CAD build for the part. Positions are in the model's coordinates, mm. Face numbers are marked on the shaded views. A direction names the side the tool comes from. Round coordinates to 2 decimals unless told otherwise and drop trailing zeros. Loops run counter-clockwise (first coordinate to the right, second up) from the corner with the lowest first, then second, coordinate; pieces in that order, holes last. Notation, with made-up numbers: (26.5, 27) - (34.5, 27) arc R25 ccw to (34.5, 65) - close; hole circle Ø1 at (81, 88.5). An arc over 180 degrees is marked (long way). One line per question, with ' | ' between items.
```python
from build123d import *

# Parameters (mm, degrees)
SKETCH2_W           = 200
SKETCH2_H           = 100
SKETCH2_W_2         = 190
SKETCH2_H_2         = 90
SKETCH2_W_3         = 65.966934908
SKETCH2_H_3         = 42.5
BOSS_EXTRUDE1_DEPTH = 5
SKETCH4_W           = 200
SKETCH4_H           = 100
SKETCH4_W_2         = 190
SKETCH4_H_2         = 90
BOSS_EXTRUDE2_DEPTH = 90
SKETCH5_W           = 70
SKETCH5_H           = 22.5
CUT_EXTRUDE1_DEPTH  = 90
SKETCH6_W           = 70
SKETCH6_H           = 22.5
CUT_EXTRUDE2_DEPTH  = 90
SKETCH7_W           = 40
SKETCH7_H           = 70
CUT_EXTRUDE3_DEPTH  = 10
SKETCH8_W           = 40
SKETCH8_H           = 70
CUT_EXTRUDE4_DEPTH  = 10
SKETCH9_W           = 40
SKETCH9_H           = 70
CUT_EXTRUDE5_DEPTH  = 10
SKETCH10_R          = 2
CUT_EXTRUDE6_DEPTH  = 10
SKETCH11_R          = 5
CUT_EXTRUDE7_DEPTH  = 150
SKETCH12_R          = 5
CUT_EXTRUDE8_DEPTH  = 10
SKETCH13_R          = 5
CUT_EXTRUDE9_DEPTH  = 10
SKETCH14_R          = 5
CUT_EXTRUDE10_DEPTH = 10
SKETCH16_R          = 0.2
CUT_EXTRUDE11_DEPTH = 10
SKETCH17_W          = 40
SKETCH17_H          = 5
BOSS_EXTRUDE3_DEPTH = 70
SKETCH18_W          = 40
SKETCH18_H          = 5
BOSS_EXTRUDE4_DEPTH = 70


with BuildPart() as part:
    # Sketch2 → Boss-Extrude1 (new body)
    with BuildSketch(Plane.XY):
        Rectangle(SKETCH2_W, SKETCH2_H)
        Rectangle(SKETCH2_W_2, SKETCH2_H_2, mode=Mode.SUBTRACT)
        Polygon((-29.033065092, -2.5), (-29.033065092, -45), (95, -45), (95, 45), (-29.033065092, 45), (-29.033065092, 2.5), (-95, 2.5), (-95, -2.5), align=None)
        with Locations((-62.016532546, -23.75)):
            Rectangle(SKETCH2_W_3, SKETCH2_H_3)
        with Locations((-62.016532546, 23.75)):
            Rectangle(SKETCH2_W_3, SKETCH2_H_3)
    extrude(amount=BOSS_EXTRUDE1_DEPTH)

    # Sketch4 → Boss-Extrude2 (add)
    with BuildSketch(Plane(origin=(0, 0, 0), x_dir=(-1, 0, 0), z_dir=(0, 0, -1))):
        Rectangle(SKETCH4_W, SKETCH4_H)
        Rectangle(SKETCH4_W_2, SKETCH4_H_2, mode=Mode.SUBTRACT)
        Polygon((30, -45), (35, -45), (35, -2.5), (95, -2.5), (95, 2.5), (35, 2.5), (35, 45), (30, 45), (30, 2.5), (-30, 2.5), (-30, 45), (-35, 45), (-35, 2.5), (-95, 2.5), (-95, -2.5), (-35, -2.5), (-35, -45), (-30, -45), (-30, -2.5), (30, -2.5), align=None)
    extrude(amount=BOSS_EXTRUDE2_DEPTH)

    # Sketch5 → Cut-Extrude1 (cut)
    with BuildSketch(Plane.ZY.offset(35)):
        with Locations((-45, 23.75)):
            Rectangle(SKETCH5_W, SKETCH5_H)
    extrude(amount=-CUT_EXTRUDE1_DEPTH, mode=Mode.SUBTRACT)

    # Sketch6 → Cut-Extrude2 (cut)
    with BuildSketch(Plane.ZY.offset(35)):
        with Locations((-45, -23.75)):
            Rectangle(SKETCH6_W, SKETCH6_H)
    extrude(amount=-CUT_EXTRUDE2_DEPTH, mode=Mode.SUBTRACT)

    # Sketch7 → Cut-Extrude3 (cut)
    with BuildSketch(Plane(origin=(0, -2.5, 0), x_dir=(-1, 0, 0), z_dir=(0, -1, 0))):
        with Locations((65, 45)):
            Rectangle(SKETCH7_W, SKETCH7_H)
    extrude(amount=-CUT_EXTRUDE3_DEPTH, mode=Mode.SUBTRACT)

    # Sketch8 → Cut-Extrude4 (cut)
    with BuildSketch(Plane(origin=(0, -2.5, 0), x_dir=(-1, 0, 0), z_dir=(0, -1, 0))):
        with Locations((0, 45)):
            Rectangle(SKETCH8_W, SKETCH8_H)
    extrude(amount=-CUT_EXTRUDE4_DEPTH, mode=Mode.SUBTRACT)

    # Sketch9 → Cut-Extrude5 (cut)
    with BuildSketch(Plane(origin=(0, -2.5, 0), x_dir=(-1, 0, 0), z_dir=(0, -1, 0))):
        with Locations((-65, 45)):
            Rectangle(SKETCH9_W, SKETCH9_H)
    extrude(amount=-CUT_EXTRUDE5_DEPTH, mode=Mode.SUBTRACT)

    # Sketch10 → Cut-Extrude6 (cut)
    with BuildSketch(Plane(origin=(0, 0, -90), x_dir=(-1, 0, 0), z_dir=(0, 0, -1))):
        with Locations((32.5, 0)):
            Circle(SKETCH10_R)
        with Locations((97.5, -47.5)):
            Circle(SKETCH10_R)
        with Locations(Location((97.5, 47.5, 0), (0, 0, 180))):
            Circle(SKETCH10_R)
        with Locations((-97.5, 47.5)):
            Circle(SKETCH10_R)
        with Locations(Location((-32.5, 0, 0), (0, 0, 180))):
            Circle(SKETCH10_R)
        with Locations(Location((-97.5, -47.5, 0), (0, 0, 180))):
            Circle(SKETCH10_R)
    extrude(amount=-CUT_EXTRUDE6_DEPTH, mode=Mode.SUBTRACT)

    # Sketch11 → Cut-Extrude7 (cut)
    with BuildSketch(Plane(origin=(0, -50, 0), x_dir=(-1, 0, 0), z_dir=(0, -1, 0))):
        with Locations(Location((60, 45, 0), (0, 0, 90))):
            Circle(SKETCH11_R)
        with Locations(Location((-60, 45, 0), (0, 0, 90))):
            Circle(SKETCH11_R)
    extrude(amount=-CUT_EXTRUDE7_DEPTH, mode=Mode.SUBTRACT)

    # Sketch12 → Cut-Extrude8 (cut)
    with BuildSketch(Plane.ZY.offset(100)):
        with Locations(Location((-42.5, -35, 0), (0, 0, 270))):
            Circle(SKETCH12_R)
    extrude(amount=-CUT_EXTRUDE8_DEPTH, mode=Mode.SUBTRACT)

    # Sketch13 → Cut-Extrude9 (cut)
    with BuildSketch(Plane(origin=(100, 0, 0), x_dir=(0, 0, -1), z_dir=(1, 0, 0))):
        with Locations(Location((42.5, -35, 0), (0, 0, 270))):
            Circle(SKETCH13_R)
    extrude(amount=-CUT_EXTRUDE9_DEPTH, mode=Mode.SUBTRACT)

    # Sketch14 → Cut-Extrude10 (cut)
    with BuildSketch(Plane.XY.offset(5)):
        with Locations((-70, -20)):
            Circle(SKETCH14_R)
        with Locations((70, -20)):
            Circle(SKETCH14_R)
    extrude(amount=-CUT_EXTRUDE10_DEPTH, mode=Mode.SUBTRACT)

    # Sketch16 → Cut-Extrude11 (cut)
    with BuildSketch(Plane.XZ.offset(50)):
        with Locations(Location((90, -5, 0), (0, 0, 270))):
            Circle(SKETCH16_R)
        with Locations(Location((91.7083249, -6.825274236, 0), (0, 0, 270))):
            Circle(SKETCH16_R)
        with Locations(Location((88.2916751, -3.174725764, 0), (0, 0, 270))):
            Circle(SKETCH16_R)
        with Locations(Location((-91.7083249, -6.825274236, 0), (0, 0, 270))):
            Circle(SKETCH16_R)
        with Locations(Location((-90, -5, 0), (0, 0, 270))):
            Circle(SKETCH16_R)
        with Locations(Location((-88.2916751, -3.174725764, 0), (0, 0, 270))):
            Circle(SKETCH16_R)
        with Locations(Location((88.2916751, -86.825274236, 0), (0, 0, 270))):
            Circle(SKETCH16_R)
        with Locations(Location((90, -85, 0), (0, 0, 270))):
            Circle(SKETCH16_R)
        with Locations(Location((91.7083249, -83.174725764, 0), (0, 0, 270))):
            Circle(SKETCH16_R)
        with Locations(Location((-88.2916751, -86.825274236, 0), (0, 0, 270))):
            Circle(SKETCH16_R)
        with Locations(Location((-90, -85, 0), (0, 0, 270))):
            Circle(SKETCH16_R)
        with Locations(Location((-91.7083249, -83.174725764, 0), (0, 0, 270))):
            Circle(SKETCH16_R)
    extrude(amount=-CUT_EXTRUDE11_DEPTH, mode=Mode.SUBTRACT)

    # Sketch17 → Boss-Extrude3 (add)
    with BuildSketch(Plane(origin=(0, 0, -10), x_dir=(-1, 0, 0), z_dir=(0, 0, -1))):
        with Locations((65, 0)):
            Rectangle(SKETCH17_W, SKETCH17_H)
    extrude(amount=BOSS_EXTRUDE3_DEPTH)

    # Sketch18 → Boss-Extrude4 (add)
    with BuildSketch(Plane(origin=(0, 0, -10), x_dir=(-1, 0, 0), z_dir=(0, 0, -1))):
        with Locations((-65, 0)):
            Rectangle(SKETCH18_W, SKETCH18_H)
    extrude(amount=BOSS_EXTRUDE4_DEPTH)


solid = part.part
```
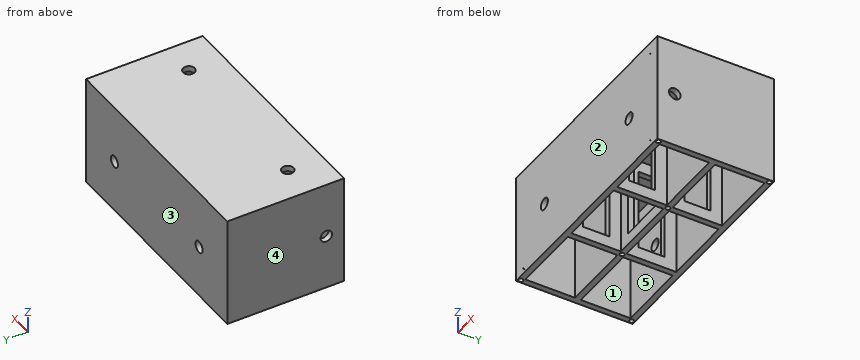
(1) Cut at B-B, the plane y = -20. State how many separate pieces and enclosed holes the cut face has, then the cut area to 3 significant figures.
Results found:
separate pieces: 5 | enclosed holes: 0 | area: 2,000 mm²
(2) Cut at D-D, the plane x = 69.5. Write the cut outline in (y, z), then the cut area to 3 significant figures.
Results found:
outline: (-50, -90) - (-45, -90) - (-45, 0) - (-24.97, 0) - (-24.97, 5) - (-50, 5) - close; (-15.03, 0) - (-2.5, 0) - (-2.5, -90) - (2.5, -90) - (2.5, 0) - (45, 0) - (45, -90) - (50, -90) - (50, 5) - (-15.03, 5) - close | area: 1,800 mm²
(3) Drop a flat-ended pin along its axis: P1, Ø6, axis at x = 39.5, y = -15, coming from the -Z side. Give the stop position or say it passes through.
Results found:
P1: stops at z = 0
(4) Tool access for the marked faces 1 and 2: list every direction of +Z, -Z, +X, -X, +Y, -Y with a clear straight run to the whole face (end or side of a thin tool).
Results found:
face 1: -Z | face 2: +Z, -Z, +X, -X, -Y
(5) Cut at C-C, the plane x = -97.5. Write the cut outline in (y, z).
Results found:
outline: (-50, -90) - (-49.5, -90) - (-49.5, -80) - (-45.5, -80) - (-45.5, -90) - (45.5, -90) - (45.5, -80) - (49.5, -80) - (49.5, -90) - (50, -90) - (50, 5) - (-50, 5) - close; hole circle Ø10 at (-35, -42.5)
(6) Probe L1, parallel to X at y = 36.5, z = -3; L2, parallel to Y at x = 15.5, z = -6; L3, parallel to X at y = -46.4, z = -45. List the from-to ranges inside material, lowest first.
Results found:
L1: x = -100 to -95, -35 to -30, 30 to 35, 95 to 100 | L2: y = -50 to -45, -2.5 to 2.5, 45 to 50 | L3: x = -100 to -65, -55 to 55, 65 to 100
(7) Two-plate mould, pull along Y, no slides. Class the marked faces 3, 4 and 5: released by +Y, released by -Y, zero draft, split by the parting line, or undercut.
Results found:
face 3: released by +Y | face 4: zero draft | face 5: undercut
(8) Cut at A-A, the plane y = 29. Write the cut outline in (x, z).
Results found:
outline: (-100, -90) - (-95, -90) - (-95, 0) - (-35, 0) - (-35, -10) - (-30, -10) - (-30, 0) - (30, 0) - (30, -10) - (35, -10) - (35, 0) - (95, 0) - (95, -90) - (100, -90) - (100, 5) - (-100, 5) - close; (-35, -90) - (-30, -90) - (-30, -80) - (-35, -80) - close; (30, -90) - (35, -90) - (35, -80) - (30, -80) - close
